from build123d import *

# Parameters (mm, degrees)
BOSS_EXTRUDE1_DEPTH           = 60
SKETCH2_W                     = 21
SKETCH2_H                     = 2
CUT_EXTRUDE1_DEPTH            = 88.893401345
CSK_FOR_M4_SFHCS1_D           = 4.5
CSK_FOR_M4_SFHCS1_CSINK_D     = 8.96
CSK_FOR_M4_SFHCS1_CSINK_ANGLE = 90


with BuildPart() as part:
    # Sketch1 → Boss-Extrude1 (new body)
    with BuildSketch(Plane(origin=(0, 0, 0), x_dir=(0, 0, -1), z_dir=(1, 0, 0))):
        Polygon((-31.5, 12.5), (-31.5, -12.5), (31.5, -12.5), (31.5, 12.5), (25.5, 12.5), (25.5, -6.5), (-25.5, -6.5), (-25.5, 12.5), align=None)
    extrude(amount=BOSS_EXTRUDE1_DEPTH)

    # Sketch2 → Cut-Extrude1 (cut, through all)
    with BuildSketch(Plane.XY.offset(31.5)):
        with Locations((30, -11.5)):
            Rectangle(SKETCH2_W, SKETCH2_H)
    extrude(amount=-CUT_EXTRUDE1_DEPTH, mode=Mode.SUBTRACT)

    # CSK for M4 SFHCS1 (through all)
    with Locations(Plane(origin=(0, -6.5, 0), x_dir=(1, 0, 0), z_dir=(0, 1, 0))):
        with Locations((10, 0), (50, 0)):
            CounterSinkHole(CSK_FOR_M4_SFHCS1_D / 2, CSK_FOR_M4_SFHCS1_CSINK_D / 2, counter_sink_angle=CSK_FOR_M4_SFHCS1_CSINK_ANGLE)


solid = part.part
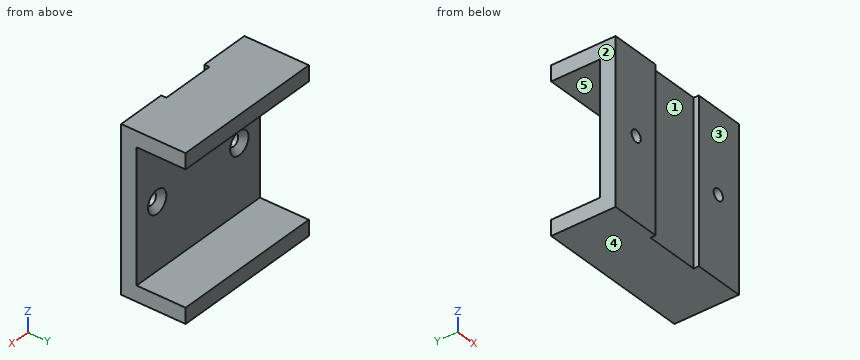
CAD build for the part. Positions are in the model's coordinates, mm. Face numbers are marked on the shaded views. A direction names the side the tool comes from. Round coordinates to 2 decimals unless told otherwise and drop trailing zeros. Write each loop counter-clockwise with the first axis right and the second up, starting at its lowest first coordinate (ties: lowest second). Pieces come first, ordered by that corner, then holes.
(1) Mould opens along X. For the marked faces 1, 2 and 3 say: pulls with the +X half, pulls with the -X half, needs draft (parallel to the pull), parting line crosses it, or undercut.
(2) 3-axis set-ups, long thin cutter, end or side, ignore diameter. For the marked faces 4 and 5: which of +Z, -Z, +X, -X, +Y, -Y reach the whole face in a straight line?
(3) Probe line 1 along Z through (x, y) = (10, -10.9); line 2 along Z through (x, y) = (23, 7); line 3 along X through (y, z) = (-11, -14). List the from-to ranges inside material, lowest first.
(4) Slice it at A-A, the plane x = 10. Write the cut outline in (y, z).
(5) Slice it at C-C, the plane z = 0. Write the cut outline in (x, y), and give its area (3 significant figures).
(6) Slice it at D-D, the plane x = 20.5. Write the cut outline in (y, z).
(7) Drop flat-ended pins along their axis: P1, Ø10.5, axis at x = 29, z = 4, coming from the -Y side; P2, Ø2.5, axis at x = 10, z = 0, coming from the -Y side. Give the stop position or say it passes through.
(8) Slice it at B-B, the plane y = -0.5. Write the cut outline in (x, z), and give its area (3 significant figures).
From the geometry:
1. face 1: undercut
1. face 2: pulls with the -X half
1. face 3: needs draft
2. face 4: -Z, +X, -X, +Y, -Y
2. face 5: +X, -X, +Y
3. line 1: z = -31.5 to -2.25, 2.25 to 31.5
3. line 2: z = -31.5 to -25.5, 25.5 to 31.5
3. line 3: x = 0 to 19.5, 40.5 to 60
4. outline: (-12.5, -31.5) - (12.5, -31.5) - (12.5, -25.5) - (-6.5, -25.5) - (-6.5, -4.48) - (-8.73, -2.25) - (-12.5, -2.25) - close; (-12.5, 2.25) - (-8.73, 2.25) - (-6.5, 4.48) - (-6.5, 25.5) - (12.5, 25.5) - (12.5, 31.5) - (-12.5, 31.5) - close
5. outline: (0, -12.5) - (7.75, -12.5) - (7.75, -8.73) - (5.52, -6.5) - (0, -6.5) - close; (12.25, -12.5) - (19.5, -12.5) - (19.5, -10.5) - (40.5, -10.5) - (40.5, -12.5) - (47.75, -12.5) - (47.75, -8.73) - (45.52, -6.5) - (14.48, -6.5) - (12.25, -8.73) - close; (52.25, -12.5) - (60, -12.5) - (60, -6.5) - (54.48, -6.5) - (52.25, -8.73) - close
5. area: 254 mm2
6. outline: (-10.5, -31.5) - (12.5, -31.5) - (12.5, -25.5) - (-6.5, -25.5) - (-6.5, 25.5) - (12.5, 25.5) - (12.5, 31.5) - (-10.5, 31.5) - close
7. P1: stops at y = -10.5
7. P2: passes through
8. outline: (0, -31.5) - (60, -31.5) - (60, -25.5) - (0, -25.5) - close; (0, 25.5) - (60, 25.5) - (60, 31.5) - (0, 31.5) - close
8. area: 720 mm2
